The listing builds one solid part. Answer for the finished solid, in the listing's coordinates (mm). A direction names the side the tool comes from. Give positions to 0.01 mm unless a question says otherwise; leave off trailing zeros. Order: outer loops, then holes, each group sorted by start corner. A loop starts at its lowest first (then second) coordinate and runs counter-clockwise, first axis right, second up.
```python
from build123d import *

# Parameters (mm, degrees)
BOSS_SWITCHMAIN_DEPTH           = 3
SKETCH1_W                       = 6.582729781
SKETCH1_H                       = 1.5
SKETCH1_W_2                     = 4.49100728
BOSS_FLANGE_WIDTH_DEPTH         = 6
SKETCH2_W                       = 5
SKETCH2_H                       = 1.490135464
SKETCH2_H_2                     = 1.5
SKETCH2_H_3                     = 2.286069733
BOSS_FLANGE_HEIGHT_DEPTH        = 11.6675
TAP_DRILL_FOR_M2X0_4_TAP1_D     = 1.6
M2_CLEARANCE_HOLE2_D            = 2.4
M2_CLEARANCE_HOLE2_DEPTH        = 6.484923868
M2_CLEARANCE_HOLE2_TIP          = 0.721032743
CUT_FLANGE_RAMP_CLEARANCE_REACH = 21.921
SKETCH10_W                      = 1.51157113
SKETCH10_H                      = 3
CUT_EXTRUDE1_REACH              = 29.069
CUT_EXTRUDE2_REACH              = 24.401
SKETCH14_W                      = 3.00210875
SKETCH14_H                      = 3.681985306
SKETCH15_W                      = 18.424052467
SKETCH15_H                      = 20.375612782
CUT_EXTRUDE3_DEPTH              = 7


with BuildPart() as part:
    # Sketch-SwitchBossUp → Boss-SwitchMain (new body)
    with BuildSketch(Plane.XY):
        with BuildLine():
            Line((6.540476927, 22.165014537), (6.540476927, 25.093856925))
            Line((6.540476927, 25.093856925), (8.540476927, 25.093856925))
            Line((8.540476927, 25.093856925), (8.540476927, 20.473554675))
            Line((8.540476927, 20.473554675), (2.463355023, 19.450530066))
            Line((2.463355023, 19.450530066), (3.558499615, 12.944990388))
            Line((3.558499615, 12.944990388), (3.581088316, 12.944953207))
            ThreePointArc((3.581088316, 12.944953207), (4.256080915, 13.944958203), (3.581073513, 14.944953207))
            Line((3.581073513, 14.944953207), (3.581073513, 17.94496801))
            Line((3.581073513, 17.94496801), (6.811292922, 17.94496801))
            Line((6.811292922, 17.94496801), (16.828083018, 17.94496801))
            Line((16.828083018, 17.94496801), (16.828083018, -1.975613284))
            Line((16.828083018, -1.975613284), (5.040476927, -1.975613284))
            Line((5.040476927, -1.975613284), (-1.954752854, -1.975613284))
            Line((-1.954752854, -1.975613284), (-1.954752854, 4.509310584))
            Line((-1.954752854, 4.509310584), (2.874043973, 4.509310584))
            Line((2.874043973, 4.509310584), (3.58114552, 5.216422599))
            ThreePointArc((3.58114552, 5.216422599), (4.256138119, 6.216427595), (3.581130717, 7.216422599))
            Line((3.581130717, 7.216422599), (2.603418204, 8.548280984))
            ThreePointArc((2.603418204, 8.548280984), (2.363042898, 9.20714873), (2.514052348, 9.892045174))
            ThreePointArc((2.514052348, 9.892045174), (2.58326881, 10.772563057), (1.97126394, 11.409393254))
            Line((1.97126394, 11.409393254), (0.5326123, 12.848023597))
            Line((0.5326123, 12.848023597), (-0.388805291, 18.321564484))
            ThreePointArc((-0.388805291, 18.321564484), (-0.224136417, 19.087558912), (0.421628056, 19.531238467))
            Line((0.421628056, 19.531238467), (-0.465233701, 24.799505683))
            ThreePointArc((-0.465233701, 24.799505683), (-2.406587703, 25.978955839), (-3.001107523, 28.171329943))
            ThreePointArc((-3.001107523, 28.171329943), (-2.220760115, 28.789797628), (-1.602292431, 28.009450221))
            ThreePointArc((-1.602292431, 28.009450221), (0.141134159, 26.168671513), (1.647974165, 28.207650602))
            ThreePointArc((1.647974165, 28.207650602), (2.167041147, 29.057364566), (3.016755111, 28.538297585))
            ThreePointArc((3.016755111, 28.538297585), (2.839798095, 26.578800421), (1.507016259, 25.131514861))
            Line((1.507016259, 25.131514861), (2.131345845, 21.422780026))
            Line((2.131345845, 21.422780026), (6.540476927, 22.165014537))
        make_face()
        with BuildLine():
            Line((5.581088316, 12.94496801), (5.581094877, 12.05857133))
            Line((5.581094877, 12.05857133), (3.97126394, 11.409408058))
            ThreePointArc((3.97126394, 11.409408058), (3.296271341, 10.409403061), (3.971278743, 9.409408058))
            Line((3.971278743, 9.409408058), (5.332971639, 10.409021979))
            Line((5.332971639, 10.409021979), (6.133921896, 10.409027907))
            Line((6.133921896, 10.409027907), (6.935397893, 9.518898634))
            Line((6.935397893, 9.518898634), (6.935397893, 8.210600129))
            Line((6.935397893, 8.210600129), (5.581130717, 7.216437402))
            ThreePointArc((5.581130717, 7.216437402), (4.906138119, 6.216432406), (5.58114552, 5.216437402))
            Line((5.58114552, 5.216437402), (6.327120808, 4.470473157))
            Line((6.327120808, 4.470473157), (6.327120808, 3.690267188))
            Line((6.327120808, 3.690267188), (5.040476927, 2.947422997))
            Line((5.040476927, 2.947422997), (5.040476927, 1.024386716))
            Line((5.040476927, 1.024386716), (8.706762674, 1.024386716))
            Line((8.706762674, 1.024386716), (10.828083018, 3.145707059))
            Line((10.828083018, 3.145707059), (10.828083018, 12.823647666))
            Line((10.828083018, 12.823647666), (8.706762674, 14.94496801))
            Line((8.706762674, 14.94496801), (6.811292922, 14.94496801))
            Line((6.811292922, 14.94496801), (5.581073513, 14.94496801))
            ThreePointArc((5.581073513, 14.94496801), (4.906080915, 13.944963014), (5.581088316, 12.94496801))
        make_face(mode=Mode.SUBTRACT)
    extrude(amount=BOSS_SWITCHMAIN_DEPTH)

    # Sketch1 → Boss-Flange Width (add)
    with BuildSketch(Plane(origin=(0, 0, 0), x_dir=(-1, 0, 0), z_dir=(0, 0, -1))):
        with Locations((-1.336612037, -0.439543551)):
            Rectangle(SKETCH1_W, SKETCH1_H)
        Polygon((-3.581073513, 17.94496801), (-6.639548057, 17.94496801), (-6.811292922, 16.454832546), (-3.581073513, 16.454832546), align=None)
        with Locations((-0.290750786, 3.759310584)):
            Rectangle(SKETCH1_W_2, SKETCH1_H)
    extrude(amount=BOSS_FLANGE_WIDTH_DEPTH)

    # Sketch2 → Boss-Flange Height (add)
    with BuildSketch(Plane(origin=(-7.039523073, 0, 0), x_dir=(0, 0, -1), z_dir=(1, 0, 0))):
        with Locations((3.5, 17.199900278)):
            Rectangle(SKETCH2_W, SKETCH2_H)
        with Locations((3.5, 3.759310584)):
            Rectangle(SKETCH2_W, SKETCH2_H_2)
        with Locations((3.5, -0.832578417)):
            Rectangle(SKETCH2_W, SKETCH2_H_3)
    extrude(amount=BOSS_FLANGE_HEIGHT_DEPTH)

    # Tap Drill for M2x0.4 Tap1 (through all)
    with Locations(Plane(origin=(0, -1.975613284, 0), x_dir=(-1, 0, 0), z_dir=(0, -1, 0))):
        with Locations((4.039523073, 3.5), (-1.627976927, 3.5)):
            Hole(TAP_DRILL_FOR_M2X0_4_TAP1_D / 2)

    # M2 Clearance Hole2
    with Locations(Plane.XZ.offset(1.975613284)):
        with Locations((-4.039523073, -3.5), (1.627976927, -3.5)):
            Hole(M2_CLEARANCE_HOLE2_D / 2, depth=M2_CLEARANCE_HOLE2_DEPTH)
            with Locations((0, 0, -(M2_CLEARANCE_HOLE2_DEPTH + M2_CLEARANCE_HOLE2_TIP / 2))):  # 118° drill point
                Cone(0, M2_CLEARANCE_HOLE2_D / 2, M2_CLEARANCE_HOLE2_TIP, mode=Mode.SUBTRACT)

    # Sketch10 → Cut-Flange Ramp Clearance (cut, up to next)
    with BuildSketch(Plane(origin=(0, 17.94496801, 0), x_dir=(1, 0, 0), z_dir=(0, 1, 0)), mode=Mode.PRIVATE) as cut_flange_ramp_clearance_sk1:
        with Locations((5.883762492, 4.5)):
            Rectangle(SKETCH10_W, SKETCH10_H)
    cut_flange_ramp_clearance_tool1 = extrude(cut_flange_ramp_clearance_sk1.sketch, amount=-CUT_FLANGE_RAMP_CLEARANCE_REACH, mode=Mode.PRIVATE) & part.part
    add(cut_flange_ramp_clearance_tool1.solids().sort_by_distance((5.883762, 17.944968, -4.5))[0], mode=Mode.SUBTRACT)

    # Sketch12 → Cut-Extrude1 (cut, up to next)
    with BuildSketch(Plane(origin=(0, 25.093856925, 0), x_dir=(1, 0, 0), z_dir=(0, 1, 0)), mode=Mode.PRIVATE) as cut_extrude1_sk1:
        Polygon((6.540476927, 0), (8.540476927, -3), (8.540476927, 0), align=None)
    cut_extrude1_tool1 = extrude(cut_extrude1_sk1.sketch, amount=-CUT_EXTRUDE1_REACH, mode=Mode.PRIVATE) & part.part
    add(cut_extrude1_tool1.solids().sort_by_distance((7.87381, 25.093857, 1))[0], mode=Mode.SUBTRACT)

    # Sketch14 → Cut-Extrude2 (cut, up to next)
    with BuildSketch(Plane(origin=(7.097281825, 8.517301779, -1.894873399), x_dir=(-0.775775184, 0.615950427, -0.137032608), z_dir=(-0.631009401, -0.757261389, 0.168470544)), mode=Mode.PRIVATE) as cut_extrude2_sk1:
        with Locations((1.064245886, -3.532126158)):
            Rectangle(SKETCH14_W, SKETCH14_H)
    cut_extrude2_tool1 = extrude(cut_extrude2_sk1.sketch, amount=-CUT_EXTRUDE2_REACH, mode=Mode.PRIVATE) & part.part
    add(cut_extrude2_tool1.solids().sort_by_distance((6.271666, 9.939876, 1.407123))[0], mode=Mode.SUBTRACT)

    # Sketch15 → Cut-Extrude3 (cut, through all)
    with BuildSketch(Plane(origin=(0, 0, 0), x_dir=(-1, 0, 0), z_dir=(0, 0, -1))):
        with Locations((-0.841389079, 8.027902003)):
            Rectangle(SKETCH15_W, SKETCH15_H)
    extrude(amount=CUT_EXTRUDE3_DEPTH, mode=Mode.SUBTRACT)


solid = part.part
```
1) A tool of negligible diameter and unlimited length cuts with its end or side. For faces 4 (the flat face through (6.54, 24, 1)), 5 (the flat face through (11, 10, 0)), 6 (the flat face through (3.581, 16, 2)), 7 (the flat face through (-0.016, 22.128, 1.479)), from which of +Z, -Z, +X, -X, +Y, -Y can it reach the whole face along a straight path? Write none if from no direction.
Geometry says:
face 4: +Z, -Z, +Y
face 5: -Z, +X, -X, +Y, -Y
face 6: +Z, -Z
face 7: +Z, -Z, -X
2) Find section C-C (x = -1). Write down the section's boundary in (y, z).
Geometry says:
outline: (-1.98, 0) - (4.51, 0) - (4.51, 3) - (-1.98, 3) - close; (24.94, 0) - (26.53, 0) - (26.53, 3) - (24.94, 3) - close
3) For a pull along Y with two mould halves and no side action, classify faces 1 (the flat face through (8, -1.976, 1)), 2 (the flat face through (-1.955, 1, 1)), 3 (the flat face through (6.71, 9.77, 2.72)) as +Y half, -Y half, draft (parallel to the pull), parting line (faces both ways), or undercut.
Geometry says:
face 1: -Y half
face 2: draft
face 3: undercut
4) Straight lines are drawn through the part: probe 1 along X at (y, z) = (8.5, 0.7); probe 2 along X at (y, z) = (14.5, 2.55); probe 3 along Y at (x, z) = (5, 0.5). For each, find the intervals that lie inside material, in ascending order.
Geometry says:
probe 1: x = 2.64 to 6.94, 10.83 to 16.83
probe 2: x = 0.25 to 3.3, 4.1 to 5.06, 9.15 to 16.83
probe 3: y = -1.98 to 5.78, 6.66 to 10.16, 11.82 to 13.5, 14.39 to 17.94, 19.88 to 21.91
5) Given P1, Ø0.6, axis at x = 7, z = 1.5, coming from the +Y side; P2, Ø0.9, axis at x = 0, z = 1, coming from the +Y side; P3, Ø5, axis at x = 4, y = 2, coming from the -Z side; P4, Ø1.5, axis at y = 0.5, z = 2, coming from the -X side, each flat-ended and moving along its own axis, determine where each tip first touches the part or whether it passes through.
Geometry says:
P1: stops at y = 25.09
P2: stops at y = 26.24
P3: stops at z = 0
P4: stops at x = -1.95
6) Find section A-A (x = 9.5). Write down the section's boundary in (y, z).
Geometry says:
outline: (-1.98, 0) - (1.82, 0) - (1.82, 3) - (-1.98, 3) - close; (14.15, 0) - (17.94, 0) - (17.94, 3) - (14.15, 3) - close
7) Find section D-D (x = 14.5). Write down the section's boundary in (y, z), then the cut area to 3 significant figures.
Geometry says:
outline: (-1.98, 0) - (17.94, 0) - (17.94, 3) - (-1.98, 3) - close
area: 59.8 mm2
8) Find section B-B (y = 24). Write down the section's boundary in (x, z).
Geometry says:
outline: (-0.33, 0) - (1.7, 0) - (1.7, 3) - (-0.33, 3) - close; (6.54, 0) - (8.54, 3) - (6.54, 3) - close
